```python
from build123d import *

# Parameters (mm, degrees)
BOSS_EXTRUDE1_DEPTH = 22.86
BOSS_EXTRUDE2_DEPTH = 12.7
FILLET1_R           = 0.3
SKETCH3_R           = 6.46557
BOSS_EXTRUDE3_DEPTH = 0.508
SKETCH4_OUTSIDE_W   = 23.02
SKETCH4_OUTSIDE_H   = 23.02
SKETCH4_OUTSIDE_R   = 4.94157
CUT_EXTRUDE1_DEPTH  = 10.16


with BuildPart() as part:
    # Sketch1 → Boss-Extrude1 (new body)
    with BuildSketch(Plane(origin=(0, 0, 0), x_dir=(1, 0, 0), z_dir=(0, 1, 0))):
        with BuildLine():
            Line((-2.68996703, 4.445), (-2.68996703, -4.445))
            ThreePointArc((-2.68996703, -4.445), (5.19557, 0), (-2.68996703, 4.445))
        make_face()
    extrude(amount=BOSS_EXTRUDE1_DEPTH)

    # Sketch2 → Boss-Extrude2 (add)
    with BuildSketch(Plane(origin=(0, 22.86, 0), x_dir=(1, 0, 0), z_dir=(0, 1, 0))):
        with BuildLine():
            Line((-1.2, -2.5), (1.2, -2.5))
            ThreePointArc((1.2, -2.5), (1.412132034, -2.412132034), (1.5, -2.2))
            Line((1.5, -2.2), (1.5, 2.2))
            ThreePointArc((1.5, 2.2), (1.412132034, 2.412132034), (1.2, 2.5))
            Line((1.2, 2.5), (-1.2, 2.5))
            ThreePointArc((-1.2, 2.5), (-1.412132034, 2.412132034), (-1.5, 2.2))
            Line((-1.5, 2.2), (-1.5, -2.2))
            ThreePointArc((-1.5, -2.2), (-1.412132034, -2.412132034), (-1.2, -2.5))
        make_face()
    extrude(amount=BOSS_EXTRUDE2_DEPTH)

    # Fillet1
    fillet1_edges = [part.edges().sort_by_distance(p)[0] for p in [
        (-1.412132034, 22.86, 2.412132034),
        (0, 22.86, 2.5),
        (1.412132034, 22.86, 2.412132034),
        (1.5, 22.86, 0),
        (1.412132034, 22.86, -2.412132034),
        (0, 22.86, -2.5),
        (-1.412132034, 22.86, -2.412132034),
        (-1.5, 22.86, 0),
    ]]
    fillet(fillet1_edges, radius=FILLET1_R)

    # Sketch3 → Boss-Extrude3 (add)
    with BuildSketch(Plane.XZ):
        Circle(SKETCH3_R)
    extrude(amount=BOSS_EXTRUDE3_DEPTH)

    # Sketch4 outside → Cut-Extrude1 (cut)
    with BuildSketch(Plane(origin=(0, 22.86, 0), x_dir=(1, 0, 0), z_dir=(0, 1, 0))):
        Rectangle(SKETCH4_OUTSIDE_W, SKETCH4_OUTSIDE_H)
        Circle(SKETCH4_OUTSIDE_R, mode=Mode.SUBTRACT)
    extrude(amount=-CUT_EXTRUDE1_DEPTH, mode=Mode.SUBTRACT)


solid = part.part
```
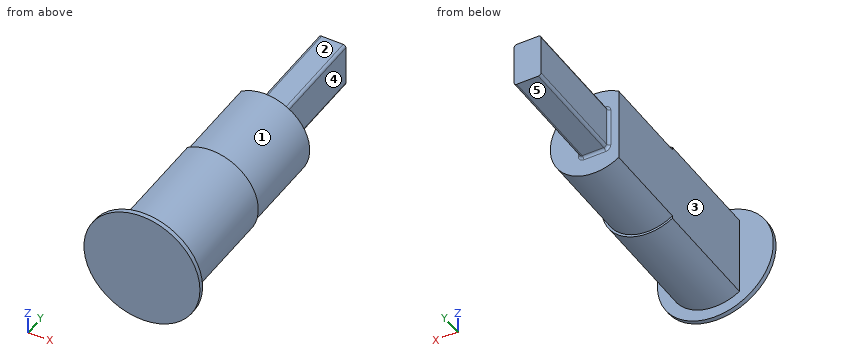
Check sheet for the modelled part. Datum: model origin and axes. Units: mm. Face numbers are marked on the shaded views. A direction names the side the tool comes from. Give positions to 0.01 mm unless a question says otherwise; leave off trailing zeros. Write each loop counter-clockwise with the first axis right and the second up, starting at its lowest first coordinate (ties: lowest second). Pieces come first, ordered by that corner, then holes. Notation, with made-up numbers: (23.25, 49.5) - (58.25, 49.5) arc R17 ccw to (58.25, 80.5) - close; hole circle Ø10 at (44.5, -3). An arc over 180 degrees is marked (long way). Answer as a JSON object with one key per item and string values. Group by question number.
1) Thickness scan on probe 1 along Y at (x, z) = (2.5, -1); probe 2 along Y at (x, z) = (0.5, -5.75); probe 3 along X at (y, z) = (32, 0.25). Record the ranges inside material, lowest first. Write a range as from..to.
2) Depth check by flat-ended pin: P1, Ø6, axis at x = 4.5, y = 9, coming from the +Z side; P2, Ø4.5, axis at y = 8, z = -1, coming from the -X side; P3, Ø2.5, axis at x = -0.5, y = 32.5, coming from the -Z side. Enter the tip coordinate at first touch or a pass-through.
3) Sectioned sample at D-D (z = 0). Record the cut outline in (x, y).
4) Sectioned sample at A-A (y = 25.5). Record the cut outline in (x, z), then the cut area to 3 significant figures.
5) Sectioned sample at B-B (z = 3.75). Record the cut outline in (x, y).
6) Access from +Z, -Z, +X, -X, +Y, -Y to the whole of each face (thin tool, end or side, straight path). Record for the marked faces 1, 2, 3, 4 and 5.
7) Sectioned sample at C-C (x = 0). Record the cut outline in (y, z), then the cut area to 3 significant figures.
Geometry results:
{
 "1": {"probe 1": "y = -0.51..22.86", "probe 2": "y = -0.51..0", "probe 3": "x = -1.5..1.5"},
 "2": {"P1": "stops at z = 4.97", "P2": "stops at x = -2.69", "P3": "stops at z = -2.5"},
 "3": {"outline": "(-6.47, -0.51) - (6.47, -0.51) - (6.47, 0) - (5.2, 0) - (5.2, 12.7) - (4.94, 12.7) - (4.94, 22.86) - (1.8, 22.86) arc R0.3 cw to (1.5, 23.16) - (1.5, 35.56) - (-1.5, 35.56) - (-1.5, 23.16) arc R0.3 cw to (-1.8, 22.86) - (-2.69, 22.86) - (-2.69, 0) - (-6.47, 0) - close"},
 "4": {"outline": "(-1.5, -2.2) arc R0.3 ccw to (-1.2, -2.5) - (1.2, -2.5) arc R0.3 ccw to (1.5, -2.2) - (1.5, 2.2) arc R0.3 ccw to (1.2, 2.5) - (-1.2, 2.5) arc R0.3 ccw to (-1.5, 2.2) - close", "area": "14.9 mm^2"},
 "5": {"outline": "(-5.27, -0.51) - (5.27, -0.51) - (5.27, 0) - (3.6, 0) - (3.6, 12.7) - (3.22, 12.7) - (3.22, 22.86) - (-2.69, 22.86) - (-2.69, 0) - (-5.27, 0) - close"},
 "6": {"face 1": "+Y", "face 2": "+Z, +X, -X, +Y", "face 3": "+Z, -Z, -X, +Y", "face 4": "+Z, -Z, +X, +Y", "face 5": "-Z, +X, -X, +Y"},
 "7": {"outline": "(-0.51, -6.47) - (0, -6.47) - (0, -5.2) - (12.7, -5.2) - (12.7, -4.94) - (22.86, -4.94) - (22.86, -2.8) arc R0.3 cw to (23.16, -2.5) - (35.56, -2.5) - (35.56, 2.5) - (23.16, 2.5) arc R0.3 cw to (22.86, 2.8) - (22.86, 4.94) - (12.7, 4.94) - (12.7, 5.2) - (0, 5.2) - (0, 6.47) - (-0.51, 6.47) - close", "area": "302 mm^2"}
}
